from build123d import *

# Parameters (mm, degrees)
SKETCH1_W           = 40
SKETCH1_H           = 50
SKETCH1_R           = 1.25
BASE_FLANGE1_DEPTH  = 2.5
SKETCH15_R          = 1
CUT_EXTRUDE3_DEPTH  = 10
JOG3_START          = -2.5
JOG3_OUTLINE_W      = 40
JOG3_OUTLINE_H      = 48.294687966
JOG3_OUTLINE_R      = 1
JOG3_OUTLINE_R_2    = 1.25
JOG3_DEPTH          = 2.5
JOG3_2_OUTLINE_W    = 40
JOG3_2_OUTLINE_H    = 1.705312034
JOG3_2_DEPTH        = 0.332528284
JOG3_START_2        = 14.2634
JOG3_3_OUTLINE_W    = 40
JOG3_3_OUTLINE_H    = 35
JOG3_3_OUTLINE_R    = 1
JOG3_3_OUTLINE_R_2  = 1.25
JOG3_3_DEPTH        = 3.2366
JOG3_4_OUTLINE_W    = 40
JOG3_4_OUTLINE_H    = 15.794687966
JOG3_4_OUTLINE_R    = 1.25
JOG3_4_DEPTH        = 3.2366
JOG3_5_OUTLINE_W    = 40
JOG3_5_OUTLINE_H    = 2.5
JOG3_5_DEPTH        = 15
JOG3_START_3        = 15
JOG3_6_OUTLINE_R    = 1.25
JOG3_6_OUTLINE_R_2  = 1
JOG3_6_DEPTH        = 2.5
JOG3_START_4        = -20
JOG3_7_DEPTH        = 40
JOG4_START          = -20
JOG4_DEPTH          = 40
JOG4_2_DEPTH        = 40
JOG4_START_2        = -3
JOG4_3_OUTLINE_R    = 1.25
JOG4_3_DEPTH        = 4
FILLET1_R           = 10
SKETCH18_R          = 2.5
BOSS_EXTRUDE1_DEPTH = 2.5
SKETCH19_R          = 1
SKETCH19_W          = 23.5
SKETCH19_H          = 12.5
CUT_EXTRUDE4_DEPTH  = 2.5
SKETCH20_R          = 2.5
SKETCH20_R_2        = 1.25
CUT_EXTRUDE6_DEPTH  = 10
SKETCH23_R          = 2.5
CUT_EXTRUDE7_DEPTH  = 44.945989578
SKETCH24_R          = 5
CUT_EXTRUDE8_DEPTH  = 1.25


with BuildPart() as part:
    # Base-Flange1: sheet metal written as solids
    # Sketch1 → Base-Flange1 (new body)
    with BuildSketch(Plane.XY):
        Rectangle(SKETCH1_W, SKETCH1_H)
        with Locations((10, 12.5)):
            Circle(SKETCH1_R, mode=Mode.SUBTRACT)
        with Locations(Location((10, -12.5, 0), (0, 0, 180))):
            Circle(SKETCH1_R, mode=Mode.SUBTRACT)
        with Locations((-10, -12.5)):
            Circle(SKETCH1_R, mode=Mode.SUBTRACT)
        with Locations(Location((-10, 12.5, 0), (0, 0, 180))):
            Circle(SKETCH1_R, mode=Mode.SUBTRACT)
    extrude(amount=-BASE_FLANGE1_DEPTH)

    # Sketch15 → Cut-Extrude3 (cut)
    with BuildSketch(Plane.XY):
        with Locations((12, 0)):
            Circle(SKETCH15_R)
        with Locations(Location((-17, 0, 0), (0, 0, 180))):
            Circle(SKETCH15_R)
    extrude(amount=-CUT_EXTRUDE3_DEPTH, mode=Mode.SUBTRACT)

    # Jog3: read off the stored shape, not the designer's step
    # Jog3 outline → Jog3 (cut)
    with BuildSketch(Plane.XY.offset(JOG3_START)):
        with Locations((0, -0.852656017)):
            Rectangle(JOG3_OUTLINE_W, JOG3_OUTLINE_H)
        with Locations((-17, 0)):
            Circle(JOG3_OUTLINE_R, mode=Mode.SUBTRACT)
        with Locations((12, 0)):
            Circle(JOG3_OUTLINE_R, mode=Mode.SUBTRACT)
        with Locations((-10, 12.5)):
            Circle(JOG3_OUTLINE_R_2, mode=Mode.SUBTRACT)
        with Locations((10, 12.5)):
            Circle(JOG3_OUTLINE_R_2, mode=Mode.SUBTRACT)
        with Locations((10, -12.5)):
            Circle(JOG3_OUTLINE_R_2, mode=Mode.SUBTRACT)
        with Locations((-10, -12.5)):
            Circle(JOG3_OUTLINE_R_2, mode=Mode.SUBTRACT)
    extrude(amount=JOG3_DEPTH, mode=Mode.SUBTRACT)

    # Jog3 2 outline → Jog3 2 (cut)
    with BuildSketch(Plane.XY.offset(JOG3_START)):
        with Locations((0, 24.147343983)):
            Rectangle(JOG3_2_OUTLINE_W, JOG3_2_OUTLINE_H)
    extrude(amount=JOG3_2_DEPTH, mode=Mode.SUBTRACT)

    # Jog3 4 outline → Jog3 4 (add)
    with BuildSketch(Plane.XY.offset(JOG3_START)):
        with Locations((0, 32.897343983)):
            Rectangle(JOG3_4_OUTLINE_W, JOG3_4_OUTLINE_H)
        with Locations((10, 28.294687966)):
            Circle(JOG3_4_OUTLINE_R, mode=Mode.SUBTRACT)
        with Locations((-10, 28.294687966)):
            Circle(JOG3_4_OUTLINE_R, mode=Mode.SUBTRACT)
    extrude(amount=JOG3_4_DEPTH)



with BuildPart() as body_2:
    # Jog3 3 outline → Jog3 3 (new body)
    with BuildSketch(Plane.XY.offset(JOG3_START_2)):
        with Locations((0, 8.294687966)):
            Rectangle(JOG3_3_OUTLINE_W, JOG3_3_OUTLINE_H)
        with Locations((12, 15.794687966)):
            Circle(JOG3_3_OUTLINE_R, mode=Mode.SUBTRACT)
        with Locations((-17, 0)):
            Circle(JOG3_3_OUTLINE_R, mode=Mode.SUBTRACT)
        with Locations((-10, 3.294687966)):
            Circle(JOG3_3_OUTLINE_R_2, mode=Mode.SUBTRACT)
        with Locations((12, 0)):
            Circle(JOG3_3_OUTLINE_R, mode=Mode.SUBTRACT)
        with Locations((10, 3.294687966)):
            Circle(JOG3_3_OUTLINE_R_2, mode=Mode.SUBTRACT)
        with Locations((-17, 15.794687966)):
            Circle(JOG3_3_OUTLINE_R, mode=Mode.SUBTRACT)
        with Locations((-10, 12.5)):
            Circle(JOG3_3_OUTLINE_R_2, mode=Mode.SUBTRACT)
        with Locations((10, 12.5)):
            Circle(JOG3_3_OUTLINE_R_2, mode=Mode.SUBTRACT)
    extrude(amount=JOG3_3_DEPTH)


with BuildPart() as part_1:
    add(part.part)

    add(body_2.part)  # Jog3 5 merges body 2
    # Jog3 5 outline → Jog3 5 (add)
    with BuildSketch(Plane.XY):
        with Locations((0, 24.544687966)):
            Rectangle(JOG3_5_OUTLINE_W, JOG3_5_OUTLINE_H)
    extrude(amount=JOG3_5_DEPTH)

    # Jog3 6 outline → Jog3 6 (add)
    with BuildSketch(Plane.XY.offset(JOG3_START_3)):
        with Locations((10, 12.5)):
            Circle(JOG3_6_OUTLINE_R)
        with Locations((-10, 12.5)):
            Circle(JOG3_6_OUTLINE_R)
        with Locations((12, 0)):
            Circle(JOG3_6_OUTLINE_R_2)
        with Locations((-17, 0)):
            Circle(JOG3_6_OUTLINE_R_2)
    extrude(amount=JOG3_6_DEPTH)

    # Jog3 7 outline → Jog3 7 (cut)
    with BuildSketch(Plane.YZ.offset(JOG3_START_4)):
        with BuildLine():
            ThreePointArc((23.294687966, 14.2634), (23.078942821, 14.784254855), (22.558087966, 15))
            Line((22.558087966, 15), (-9.205312034, 15))
            Line((-9.205312034, 15), (-9.205312034, 14.2634))
            Line((-9.205312034, 14.2634), (23.294687966, 14.2634))
        make_face()
        with BuildLine():
            ThreePointArc((26.531287966, -2.5), (24.242666158, -1.552021808), (23.294687966, 0.7366))
            Line((23.294687966, 0.7366), (23.294687966, -2.167471716))
            Line((23.294687966, -2.167471716), (25, -2.167471716))
            Line((25, -2.167471716), (25, -2.5))
            Line((25, -2.5), (26.531287966, -2.5))
        make_face()
        with BuildLine():
            Line((26.531287966, 0), (40.794687966, 0))
            Line((40.794687966, 0), (40.794687966, 0.7366))
            Line((40.794687966, 0.7366), (25.794687966, 0.7366))
            ThreePointArc((25.794687966, 0.7366), (26.010433111, 0.215745145), (26.531287966, 0))
        make_face()
        with BuildLine():
            Line((25.794687966, 17.5), (22.558087966, 17.5))
            ThreePointArc((22.558087966, 17.5), (24.846709774, 16.552021808), (25.794687966, 14.2634))
            Line((25.794687966, 14.2634), (25.794687966, 17.5))
        make_face()
    extrude(amount=JOG3_7_DEPTH, mode=Mode.SUBTRACT)

    # Jog4: read off the stored shape, not the designer's step
    # Jog4 outline → Jog4 (cut)
    with BuildSketch(Plane.YZ.offset(JOG4_START)):
        with BuildLine():
            Line((-9.205312034, 15), (5.87962174, 15))
            ThreePointArc((5.87962174, 15), (7.019882984, 16.799110859), (9.031287966, 17.5))
            Line((9.031287966, 17.5), (-9.205312034, 17.5))
            Line((-9.205312034, 17.5), (-9.205312034, 15))
        make_face()
    extrude(amount=JOG4_DEPTH, mode=Mode.SUBTRACT)

    # Jog4 2 outline → Jog4 2 (add)
    with BuildSketch(Plane.YZ.offset(JOG4_START)):
        with BuildLine():
            Line((-9.205312034, 0), (-9.205312034, -2.5))
            Line((-9.205312034, -2.5), (5.058087966, -2.5))
            ThreePointArc((5.058087966, -2.5), (7.346709774, -1.552021808), (8.294687966, 0.7366))
            Line((8.294687966, 0.7366), (8.294687966, 14.2634))
            ThreePointArc((8.294687966, 14.2634), (8.510433111, 14.784254855), (9.031287966, 15))
            Line((9.031287966, 15), (5.87962174, 15))
            ThreePointArc((5.87962174, 15), (5.81599152, 14.634140241), (5.794687966, 14.2634))
            Line((5.794687966, 14.2634), (5.794687966, 0.7366))
            ThreePointArc((5.794687966, 0.7366), (5.578942821, 0.215745145), (5.058087966, 0))
            Line((5.058087966, 0), (-9.205312034, 0))
        make_face()
    extrude(amount=JOG4_2_DEPTH)

    # Jog4 3 outline → Jog4 3 (cut)
    with BuildSketch(Plane.XY.offset(JOG4_START_2)):
        with Locations((-10, 3.294687966)):
            Circle(JOG4_3_OUTLINE_R)
        with Locations((10, 3.294687966)):
            Circle(JOG4_3_OUTLINE_R)
    extrude(amount=JOG4_3_DEPTH, mode=Mode.SUBTRACT)

    # Fillet1
    fillet1_edges = [part_1.edges().sort_by_distance(p)[0] for p in [
        (20, -9.205312034, -1.25),
        (-20, -9.205312034, -1.25),
        (-20, 40.794687966, -1.25),
        (20, 40.794687966, -1.25),
    ]]
    fillet(fillet1_edges, radius=FILLET1_R)

    # Sketch18 → Boss-Extrude1 (add)
    with BuildSketch(Plane.XY.offset(17.5)):
        with Locations((12, 15.794687966)):
            Circle(SKETCH18_R)
        with Locations((-17, 15.794687966)):
            Circle(SKETCH18_R)
    extrude(amount=-BOSS_EXTRUDE1_DEPTH)

    # Sketch19 → Cut-Extrude4 (cut)
    with BuildSketch(Plane(origin=(0, 25.794687966, 0), x_dir=(1, 0, 0), z_dir=(0, 1, 0))):
        with Locations(Location((13.9, -7.5, 0), (0, 0, 270))):
            Circle(SKETCH19_R)
        with Locations(Location((-13.9, -7.5, 0), (0, 0, 90))):
            Circle(SKETCH19_R)
        with Locations((0, -7.5)):
            Rectangle(SKETCH19_W, SKETCH19_H)
    extrude(amount=-CUT_EXTRUDE4_DEPTH, mode=Mode.SUBTRACT)

    # Sketch20 → Cut-Extrude6 (cut)
    with BuildSketch(Plane.XY):
        with Locations((0, 33.294687966)):
            Circle(SKETCH20_R)
        with Locations(Location((0, -1.705312034, 0), (0, 0, 180))):
            Circle(SKETCH20_R)
        with Locations((7.5, -1.705312034)):
            Circle(SKETCH20_R_2)
        with Locations(Location((-7.5, -1.705312034, 0), (0, 0, 180))):
            Circle(SKETCH20_R_2)
        with Locations(Location((7.5, 33.294687966, 0), (0, 0, 180))):
            Circle(SKETCH20_R_2)
        with Locations((-7.5, 33.294687966)):
            Circle(SKETCH20_R_2)
    extrude(amount=-CUT_EXTRUDE6_DEPTH, mode=Mode.SUBTRACT)

    # Sketch23 → Cut-Extrude7 (cut, through all)
    with BuildSketch(Plane(origin=(0, 25.794687966, 0), x_dir=(1, 0, 0), z_dir=(0, 1, 0))):
        with Locations(Location((-5.55, -7.5, 0), (0, 0, 270))):
            Circle(SKETCH23_R)
    extrude(amount=-CUT_EXTRUDE7_DEPTH, mode=Mode.SUBTRACT)

    # Sketch24 → Cut-Extrude8 (cut)
    with BuildSketch(Plane(origin=(0, 8.294687966, 0), x_dir=(1, 0, 0), z_dir=(0, 1, 0))):
        with Locations(Location((-5.55, -7.5, 0), (0, 0, 270))):
            Circle(SKETCH24_R)
    extrude(amount=-CUT_EXTRUDE8_DEPTH, mode=Mode.SUBTRACT)


solid = part_1.part
Can you work these out from the model? Positions are in its coordinate system, mm. A direction names the side the tool comes from. Give positions to 0.01 mm unless a question says otherwise; leave off trailing zeros. Order: outer loops, then holes, each group sorted by start corner. A loop starts at its lowest first (then second) coordinate and runs counter-clockwise, first axis right, second up. Notation, with made-up numbers: M 7.5,-15.75 L 26.5,-15.75 A24 cw 26.5,6.25 Z; hole C 26,-35.75 d10. An arc over 180 degrees is marked long. Use a Markdown table: item, result. Add a question column.
Item 1: Suppose I cut it at A-A (x = 0). Count the separate pieces of the cut face and the enclosed holes in it, then the cut area to 3 significant figures.
Item 2: We'd pull the mould along Z, two halves only. Please class faces 1 (the cylindrical face through (-0.3, 24.8, 16.6)), 2 (the cylindrical face through (-16.993, -6.354, -1.268)), 3 (the flat face through (0, 25, 1.25)): +Z half, -Z half, draft (parallel to the pull), parting line (faces both ways), or undercut.
Item 3: If I drill on L1, parallel to X at y = 24.95, z = 7.5; L2, parallel to Y at x = -5, z = 0.75; L3, parallel to Y at x = 0, z = -1.45 (3 decimals), over which ranges is the centre line in solid material (lowest first)? Write a range as [from, to].
Item 4: Suppose I cut it at C-C (x = 13.9). List the corners of the cut face in (y, z) for me.
Item 5: For faces 4 (the flat face through (11.75, 25, 8)), 5 (the flat face through (-14, 25.795, 9)), 6 (the flat face through (-14, 23.295, 9)), 7 (the flat face through (0, 1, 0)), which set-ups out of +Z, -Z, +X, -X, +Y, -Y let a thin tool reach every point of the face, with its end or its side?
Item 6: Will these pins go through, and if not, where does the flat tip stop? pin 1 (10 mm diameter, centred on x = 4.5, z = 7.5, fed in from -Y); pin 2 (8 mm diameter, centred on x = 3.5, z = 5.5, fed in from +Y); pin 3 (3 mm diameter, centred on x = -7.5, y = -1.71, fed in from +Z).
Item 7: Suppose I cut it at B-B (z = 7.5). List the corners of the cut face in (x, y) for me.
Answer sheet:
| question | item | result |
|---|---|---|
| 1 | separate pieces | 4 |
| 1 | enclosed holes | 0 |
| 1 | area | 148 mm² |
| 2 | face 1 | +Z half |
| 2 | face 2 | draft |
| 2 | face 3 | undercut |
| 3 | L1 | x = [-20, -14.9], [-12.9, -11.75], [11.75, 12.9], [14.9, 20] |
| 3 | L2 | y = [5.79, 8.29], [23.29, 25.79] |
| 3 | L3 | y = [-9.205, -4.205], [0.795, 7.444], [24.145, 30.795], [35.795, 40.795] |
| 4 | outline | M -8.41,-2.5 L 5.06,-2.5 A3.24 ccw 8.29,0.74 L 8.29,14.26 A0.74 cw 9.03,15 L 22.56,15 A0.74 cw 23.29,14.26 L 23.29,8.5 L 25.79,8.5 L 25.79,14.26 A3.24 ccw 22.56,17.5 L 9.03,17.5 A3.24 ccw 5.79,14.26 L 5.79,0.74 A0.74 cw 5.06,0 L -8.41,0 Z; M 23.29,0.74 A3.24 ccw 26.53,-2.5 L 40,-2.5 L 40,0 L 26.53,0 A0.74 cw 25.79,0.74 L 25.79,6.5 L 23.29,6.5 Z |
| 5 | face 4 | +Y |
| 5 | face 5 | +Z, +X, -X, +Y |
| 5 | face 6 | -Z, +X, -X |
| 5 | face 7 | +Z, +X, -X, -Y |
| 6 | pin 1 | stops at y = 5.79 |
| 6 | pin 2 | stops at y = 8.29 |
| 6 | pin 3 | stops at z = 0 |
| 7 | outline | M -20,5.79 L -8.05,5.79 L -8.05,7.04 L -10.55,7.04 L -10.55,8.29 L -20,8.29 Z; M -20,23.29 L -14.9,23.29 L -14.9,25.79 L -20,25.79 Z; M -12.9,23.29 L -11.75,23.29 L -11.75,25.79 L -12.9,25.79 Z; M -3.05,5.79 L 20,5.79 L 20,8.29 L -0.55,8.29 L -0.55,7.04 L -3.05,7.04 Z; M 11.75,23.29 L 12.9,23.29 L 12.9,25.79 L 11.75,25.79 Z; M 14.9,23.29 L 20,23.29 L 20,25.79 L 14.9,25.79 Z |
